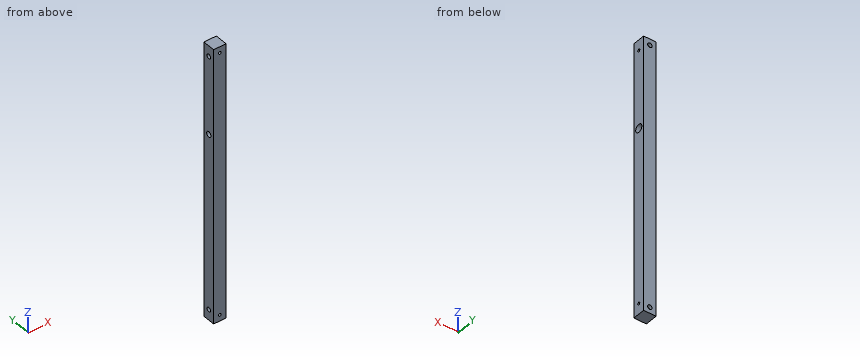
from build123d import *

# Parameters (mm, degrees)
IZIM1_W                     = 28
IZIM1_H                     = 28
Y_KSEKLIK_EKSTR_ZYON1_DEPTH = 620
IZIM3_R                     = 5
KES_EKSTR_ZYON2_DEPTH       = 7
IZIM4_R                     = 3
KES_EKSTR_ZYON3_DEPTH       = 29
IZIM5_R                     = 6
KES_EKSTR_ZYON4_DEPTH       = 29
IZIM6_R                     = 9
KES_EKSTR_ZYON5_DEPTH       = 10
KES_EKSTR_ZYON6_REACH       = 30
IZIM7_R                     = 3
IZIM9_R                     = 5
KES_EKSTR_ZYON8_DEPTH       = 7


with BuildPart() as part:
    # Çizim1 → Yükseklik-Ekstrüzyon1 (new body)
    with BuildSketch(Plane.XY):
        Rectangle(IZIM1_W, IZIM1_H)
    extrude(amount=Y_KSEKLIK_EKSTR_ZYON1_DEPTH)

    # Çizim3 → Kes-Ekstrüzyon2 (cut)
    with BuildSketch(Plane(origin=(0, 14, 0), x_dir=(1, 0, 0), z_dir=(0, 1, 0))):
        with Locations((0, -14)):
            Circle(IZIM3_R)
        with Locations((0, -606)):
            Circle(IZIM3_R)
    extrude(amount=-KES_EKSTR_ZYON2_DEPTH, mode=Mode.SUBTRACT)

    # Çizim4 → Kes-Ekstrüzyon3 (cut, through all)
    with BuildSketch(Plane(origin=(0, 14, 0), x_dir=(1, 0, 0), z_dir=(0, 1, 0))):
        with Locations((0, -606)):
            Circle(IZIM4_R)
        with Locations((0, -14)):
            Circle(IZIM4_R)
    extrude(amount=-KES_EKSTR_ZYON3_DEPTH, mode=Mode.SUBTRACT)

    # Çizim5 → Kes-Ekstrüzyon4 (cut, through all)
    with BuildSketch(Plane(origin=(14, 0, 0), x_dir=(0, 0, -1), z_dir=(1, 0, 0))):
        with Locations((-420, 0)):
            Circle(IZIM5_R)
    extrude(amount=-KES_EKSTR_ZYON4_DEPTH, mode=Mode.SUBTRACT)

    # Çizim6 → Kes-Ekstrüzyon5 (cut)
    with BuildSketch(Plane(origin=(14, 0, 0), x_dir=(0, 0, -1), z_dir=(1, 0, 0))):
        with Locations((-420, 0)):
            Circle(IZIM6_R)
    extrude(amount=-KES_EKSTR_ZYON5_DEPTH, mode=Mode.SUBTRACT)

    # Çizim7 → Kes-Ekstrüzyon6 (cut, up to next)
    with BuildSketch(Plane(origin=(14, 0, 0), x_dir=(0, 0, -1), z_dir=(1, 0, 0)), mode=Mode.PRIVATE) as kes_ekstr_zyon6_sk1:
        with Locations((-24, 0)):
            Circle(IZIM7_R)
    kes_ekstr_zyon6_tool1 = extrude(kes_ekstr_zyon6_sk1.sketch, amount=-KES_EKSTR_ZYON6_REACH, mode=Mode.PRIVATE) & part.part
    add(kes_ekstr_zyon6_tool1.solids().sort_by_distance((14, 0, 24))[0], mode=Mode.SUBTRACT)
    # Çizim7 → Kes-Ekstrüzyon6 (cut, up to next)
    with BuildSketch(Plane(origin=(14, 0, 0), x_dir=(0, 0, -1), z_dir=(1, 0, 0)), mode=Mode.PRIVATE) as kes_ekstr_zyon6_sk2:
        with Locations((-596, 0)):
            Circle(IZIM7_R)
    kes_ekstr_zyon6_tool2 = extrude(kes_ekstr_zyon6_sk2.sketch, amount=-KES_EKSTR_ZYON6_REACH, mode=Mode.PRIVATE) & part.part
    add(kes_ekstr_zyon6_tool2.solids().sort_by_distance((14, 0, 596))[0], mode=Mode.SUBTRACT)

    # Çizim9 → Kes-Ekstrüzyon8 (cut)
    with BuildSketch(Plane.ZY.offset(14)):
        with Locations((596, 0)):
            Circle(IZIM9_R)
        with Locations((24, 0)):
            Circle(IZIM9_R)
    extrude(amount=-KES_EKSTR_ZYON8_DEPTH, mode=Mode.SUBTRACT)


solid = part.part
Read the model definition and answer for the solid it produces. Units are mm, in the model's axes. Give positions to 0.01 mm unless a question says otherwise; leave off trailing zeros. Loops run counter-clockwise (first coordinate to the right, second up) from the corner with the lowest first, then second, coordinate; pieces in that order, holes last. Notation, with made-up numbers: (73.5, -20) - (84.5, -20) arc R33 cw to (84.5, 14) - close; hole circle Ø10 at (62, 48). An arc over 180 degrees is marked (long way). Answer as CSV lines item,"result". Start each with the question number.
1) Find section B-B (z = 420). Write down the section's boundary in (x, y), then the cut area to 3 significant figures.
2) Each of these flat-tipped pins is pushed along its axis until it touches: pin 1 Ø8 at (x, z) = (0, 606) entering from +Y; pin 2 Ø9.5 at (x, z) = (0, 14) entering from -Y; pin 3 Ø5 at (y, z) = (0, 24) entering from -X. Where does it stop, or does it pass through?
3) Find section A-A (x = 9.5). Write down the section's boundary in (y, z).
4) Straight lines are drawn through the part: L1, parallel to Z at x = 0, y = 11; L2, parallel to Z at x = 4, y = 10.75; L3, parallel to Z at x = -6, y = -0.25. For each, find the intervals that lie inside material, in ascending order. Write a range as from..to.
Findings below:
1,outline,"(-14, -14) - (14, -14) - (14, -9) - (4, -9) - (4, -6) - (-14, -6) - close; (-14, 6) - (4, 6) - (4, 9) - (14, 9) - (14, 14) - (-14, 14) - close"
1,area,"388 mm^2"
2,pin 1,"y = 7"
2,pin 2,"y = -14"
2,pin 3,"through"
3,outline,"(-14, 0) - (14, 0) - (14, 620) - (-14, 620) - close; hole circle Ø18 at (0, 420); hole circle Ø6 at (0, 24); hole circle Ø6 at (0, 596)"
4,L1,"0..9, 19..601, 611..620"
4,L2,"0..11, 17..603, 609..620"
4,L3,"0..21.01, 26.99..414.01, 425.99..593.01, 598.99..620"
